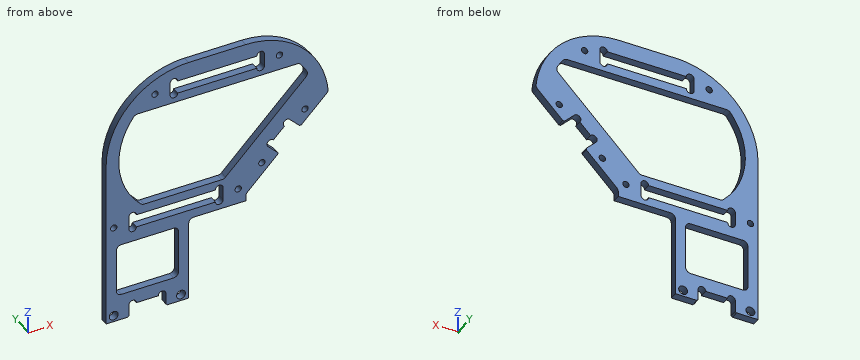
Autodesk Inventor part; units mm, degrees
ref_plane "YZ Plane" through (0, 0, 0) normal (1, 0, 0) x (0, 1, 0)
ref_plane "XZ Plane" through (0, 0, 0) normal (0, 1, 0) x (-1, 0, 0)
ref_plane "XY Plane" through (0, 0, 0) normal (0, 0, 1) x (1, 0, 0)
sketch "Sketch1" plane through (0, 0, 0) normal (0, 1, 0) x (-1, 0, 0)
  line L0 (-16.25, -1.5) -> (16.25, -1.5)
  line L1 (-7.25, -1.5) -> (-7.25, 3.5) construction
  line L2 (-7.25, 3.5) -> (7.25, 3.5) construction
  line L3 (0, 3.5) -> (0, -1.5) construction
  line L4 (7.25, -1.5) -> (7.25, 3.5) construction
  line L5 (-13.25, 1) -> (13.25, 1) construction
  line L6 (-7.3, -1.5) -> (-7.3, 3.5)
  line L7 (-7.3, 3.5) -> (7.3, 3.5)
  arc A0 (-4.3, 3.5) -> (-7.3, 3.5) centre (-5.8, 3.5) ccw
  line L8 (7.3, -1.5) -> (7.3, 3.5)
  arc A1 (7.3, 3.5) -> (4.3, 3.5) centre (5.8, 3.5) ccw
  line L9 (-16.25, -1.5) -> (-16.25, 32)
  line L10 (16.25, -1.5) -> (16.25, 65)
  ellipse E0 centre (-16.25, 65) end of major axis (18.25, 65) minor radius 35 (-16.25, 30) -> (-16.25, 100) ccw construction
  line L11 (-16.25, 30) -> (-16.25, 100) construction
  line L12 (-16.25, 65) -> (18.25, 65) construction
  ellipse E1 centre (-16.25, 65) end of major axis (16.25, 65) minor radius 33 (-16.25, 32) -> (16.25, 65) ccw construction
  line L13 (-16.25, 32) -> (-38.75, 32)
  line L14 (-16.25, 98) -> (-38.75, 98)
  line L15 (-27.5, 98) -> (-27.5, 32) construction
  ellipse E2 centre (-38.75, 65) end of major axis (-73.25, 65) minor radius 35 (-38.75, 100) -> (-38.75, 30) ccw construction
  ellipse E3 centre (-38.75, 65) end of major axis (-71.25, 65) minor radius 33 (-38.75, 98) -> (-71.1715, 67.2921) ccw
  line L16 (-38.75, 30) -> (-16.25, 30) construction
  line L17 (-38.75, 100) -> (-16.25, 100) construction
  line L18 (-10.25, 30) -> (10.25, 30)
  line L19 (12.25, 28) -> (12.25, 11)
  line L20 (10.25, 9) -> (-10.25, 9)
  line L21 (-12.25, 11) -> (-12.25, 28)
  line L22 (-12.25, 30) -> (12.25, 9) construction
  line L23 (12.25, 30) -> (-12.25, 9) construction
  arc A2 (-10.25, 30) -> (-12.25, 28) centre (-10.25, 28) ccw
  arc A3 (-12.25, 11) -> (-10.25, 9) centre (-10.25, 11) ccw
  arc A4 (10.25, 9) -> (12.25, 11) centre (10.25, 11) ccw
  arc A5 (12.25, 28) -> (10.25, 30) centre (10.25, 28) ccw
  line L24 (-38.75, 30) -> (-38.75, 100) construction
  line L25 (-38.75, 32) -> (-38.75, 34.8706)
  line L26 (-38.75, 34.8706) -> (-71.1715, 67.2921)
  line L27 (-62.0208, 45.9792) -> (-108, 0) construction
  line L28 (-108, 0) -> (0, 0) construction
  ellipse E4 centre (-38.75, 65) end of major axis (-71.25, 65) minor radius 33 (-71.1715, 67.2921) -> (-38.75, 32) ccw construction
  ellipse E5 centre (-16.25, 65) end of major axis (16.25, 65) minor radius 33 (16.25, 65) -> (-16.25, 98) ccw
  line L29 (-55, 91.5815) -> (0, 91.5815) construction
  line L30 (0, 91.5815) -> (0, 86.5815) construction
  line L31 (0, 86.5815) -> (-55, 86.5815) construction
  line L32 (-55, 86.5815) -> (-55, 91.5815) construction
  line L33 (-55, 91.5815) -> (0, 86.5815) construction
  line L34 (0, 91.5815) -> (-55, 86.5815) construction
  line L35 (-47.5, 91.5815) -> (-47.5, 96.7815) construction
  line L36 (-47.5, 96.7815) -> (-7.5, 96.7815) construction
  line L37 (-7.5, 96.7815) -> (-7.5, 91.5815) construction
  line L38 (-46, 91.5815) -> (-46, 86.5815) construction
  line L39 (-52, 89.0815) -> (-3, 89.0815) construction
  line L40 (-9, 91.5815) -> (-9, 86.5815) construction
  line L41 (-8.95, 86.5315) -> (-46.05, 86.5315)
  line L42 (-46.05, 86.5315) -> (-46.05, 91.6315)
  line L43 (-46.05, 91.6315) -> (-8.95, 91.6315)
  line L44 (-8.95, 91.6315) -> (-8.95, 86.5315)
  line L45 (-8.95, 86.5315) -> (-46.05, 91.6315) construction
  line L46 (-46.05, 86.5315) -> (-8.95, 91.6315) construction
  arc A6 (-43.05, 91.6315) -> (-46.05, 91.6315) centre (-44.55, 91.6315) ccw
  arc A7 (-46.05, 86.5315) -> (-43.05, 86.5315) centre (-44.55, 86.5315) ccw
  arc A8 (-8.95, 91.6315) -> (-11.95, 91.6315) centre (-10.45, 91.6315) ccw
  arc A9 (-11.95, 86.5315) -> (-8.95, 86.5315) centre (-10.45, 86.5315) ccw
  line L47 (-54.1012, 75.112) -> (-60.6066, 68.6066) construction
  line L48 (-60.6066, 68.6066) -> (-39.3934, 47.3934) construction
  line L49 (-39.3934, 47.3934) -> (-32.888, 53.8988) construction
  line L50 (-32.888, 53.8988) -> (-54.1012, 75.112) construction
  line L51 (-56.0104, 64.0104) -> (-72.2739, 47.747) construction
  line L52 (-72.2739, 47.747) -> (-60.253, 35.7261) construction
  line L53 (-60.253, 35.7261) -> (-43.9896, 51.9896) construction
  line L54 (-60.1823, 56.3029) -> (-56.0104, 60.4749) construction
  line L55 (-56.0104, 60.4749) -> (-47.5251, 51.9896) construction
  line L56 (-47.5251, 51.9896) -> (-51.6971, 47.8177) construction
  line L57 (-60.2177, 56.3383) -> (-56.0458, 60.5102)
  line L58 (-56.0458, 60.5102) -> (-47.4898, 51.9542)
  line L59 (-47.4898, 51.9542) -> (-51.6617, 47.7823)
  arc A10 (-47.4898, 51.9542) -> (-49.6111, 54.0756) centre (-48.5504, 53.0149) ccw
  arc A11 (-53.9244, 58.3889) -> (-56.0458, 60.5102) centre (-54.9851, 59.4496) ccw
  line L60 (-62.0208, 62.9497) -> (-45.0503, 45.9792) construction
  line L61 (-51.7678, 56.2322) -> (-55.3033, 52.6967) construction
  line L62 (-59.5459, 56.9393) -> (-51.0607, 48.4541) construction
  circle A12 centre (-45.0503, 45.9792) radius 2.4 construction
  circle A13 centre (-45.0503, 45.9792) radius 1.25 construction
  line L63 (-65.9099, 63.3033) -> (-62.3744, 66.8388) construction
  line L64 (-44.6967, 42.0901) -> (-41.1612, 45.6256) construction
  line L65 (-29.75, 40.55) -> (7.25, 40.55) construction
  line L66 (7.25, 40.55) -> (7.25, 35.55) construction
  line L67 (7.25, 35.55) -> (-29.75, 35.55) construction
  line L68 (-29.75, 35.55) -> (-29.75, 40.55) construction
  line L69 (-29.75, 40.55) -> (7.25, 35.55) construction
  line L70 (7.25, 40.55) -> (-29.75, 35.55) construction
  line L71 (-35.75, 38.05) -> (13.25, 38.05) construction
  line L72 (-11.25, 40.55) -> (-11.25, 35.55) construction
  line L73 (-38.75, 40.55) -> (-38.75, 35.55) construction
  line L74 (16.25, 40.55) -> (16.25, 35.55) construction
  line L75 (-29.8, 40.6) -> (7.3, 40.6)
  line L76 (7.3, 40.6) -> (7.3, 35.5)
  line L77 (7.3, 35.5) -> (-29.8, 35.5)
  line L78 (-29.8, 35.5) -> (-29.8, 40.6)
  line L79 (-29.8, 40.6) -> (7.3, 35.5) construction
  line L80 (7.3, 40.6) -> (-29.8, 35.5) construction
  arc A14 (4.3, 35.5) -> (7.3, 35.5) centre (5.8, 35.5) ccw
  arc A15 (7.3, 40.6) -> (4.3, 40.6) centre (5.8, 40.6) ccw
  arc A16 (-29.8, 35.5) -> (-26.8, 35.5) centre (-28.3, 35.5) ccw
  arc A17 (-26.8, 40.6) -> (-29.8, 40.6) centre (-28.3, 40.6) ccw
  line L81 (-59.7893, 83.0315) -> (4.7893, 83.0315)
  line L82 (-63.4241, 77.3638) -> (-30.1603, 44.1)
  ellipse E6 centre (-16.25, 65) end of major axis (11.25, 65) minor radius 28.0012 (2.0513, 44.1) -> (11.25, 65) ccw
  ellipse E7 centre (-16.25, 65) end of major axis (11.25, 65) minor radius 28.0012 (11.25, 65) -> (4.7893, 83.0315) ccw
  ellipse E8 centre (-38.75, 65) end of major axis (-66.25, 65) minor radius 28.0012 (-59.7893, 83.0315) -> (-63.4241, 77.3638) ccw
  line L83 (-16.25, 65) -> (8.5857, 86.2852) construction
  line L84 (-30.1603, 44.1) -> (2.0513, 44.1)
  line L85 (-62.0208, 45.9792) -> (-32.844, 9.9488)
  line L86 (-32.844, 9.9488) -> (-98.0512, 75.156)
  line L87 (-98.0512, 75.156) -> (-62.0208, 45.9792)
  line L88 (-38.75, 65) -> (-73.25, 65) construction
  point P0 (0, 1)
  point P1 (0, 19.5)
  point P2 (5.8, 5)
  point P3 (-27.5, 89.0815)
  point P4 (-53.5355, 54.4645)
  point P5 (-50, 58)
  point P6 (-11.25, 38.05)
  point P7 (-11.25, 38.05)
  point P8 (4.3, 3.5)
  point P9 (-53.9244, 58.3889)
  point P10 (-26.8, 35.5)
  point P11 (-26.8, 40.6)
  point P12 (4.3, 40.6)
  point P13 (-11.95, 91.6315)
  point P14 (-11.95, 86.5315)
  point P15 (-43.05, 86.5315)
  point P16 (-10.45, 85.0315)
  point P17 (-28.3, 34)
  point P18 (5.8, 42.1)
  point P19 (-27.5, 89.0815)
  dimension "d0" = 32.5
  dimension "d1" = 9
  dimension "d2" = 6
  dimension "d3" = 1.5
  dimension "d4" = 5
  dimension "d5" = 0.05
  dimension "d7" = 1.5
  dimension "d8" = 70
  dimension "d10" = 100
  dimension "d12" = 2
  dimension "d14" = 2
  dimension "d15" = 22.5
  dimension "d16" = 4
  dimension "d18" = 2
  dimension "d19" = 55
  dimension "d20" = 5
  dimension "d21" = 5.2
  dimension "d22" = 40
  dimension "d24" = 9
  dimension "d25" = 6
  dimension "d26" = 0.05
  dimension "d27" = 0.05
  dimension "d28" = 6
  dimension "d29" = 9.2
  dimension "d30" = 23
  dimension "d31" = 17
  dimension "d32" = 30
  dimension "d33" = 0.05
  dimension "d34" = 5
  dimension "d35" = 6
  dimension "d36" = 2.5
  dimension "d37" = 4.8
  dimension "d38" = 2.5
  dimension "d39" = 1
  dimension "d40" = 50
  dimension "d41" = 58
  dimension "d42" = 45
  dimension "d43" = 30
  dimension "d44" = 9
  dimension "d46" = 5
  dimension "d47" = 6
  dimension "d48" = 9
  dimension "d49" = 0.05
  dimension "d50" = 0.05
  dimension "d54" = 5
  dimension "d56" = 10
  dimension "d59" = 5
  dimension "d61" = 3.55
  dimension "d80" = 55
  dimension "d83" = 2
  dimension "d84" = 2
  dimension "d85" = 168
  dimension "d86" = 24.5
  dimension "d87" = 2
extrude "Extrusion1" add sketch "Sketch1" along normal blind 3 contours L9 L13 L25 L26 L59 A10 L58 A11 L57 E3 L14 E5 L10 L0 L8 A1 L7 A0 L6
hole "Phi3.5" at (13.25, 0, 1) at (-13.25, 0, 1) direction (0, 1, 0) diameter 3.5 end through all
hole "Phi2.5" at (52, 0, 89.0815) at (3, 0, 89.0815) at (62.0208, 0, 62.9497) at (45.0503, 0, 45.9792) at (35.75, 0, 38.05) at (-13.25, 0, 38.05) direction (0, 1, 0) diameter 2.5 end through all
chamfer "C0.5" distance 0.5 angle 45 4 edges at (60.2177, 1.5, 56.3383) (51.6617, 1.5, 47.7823) (7.3, 1.5, -1.5) (-7.3, 1.5, -1.5)
fillet "R2" radius 2 8 edges at (63.4241, 1.5, 77.3638) (59.7893, 1.5, 83.0315) (-4.7893, 1.5, 83.0315) (-2.0513, 1.5, 44.1) (30.1603, 1.5, 44.1) (16.25, 1.5, 32) (38.75, 1.5, 34.8706) (71.1715, 1.5, 67.2921)
equation "\"d14\" = d12"
properties part number "HeadSideFrame" material "CFRP"
The model under review builds one solid part; all positions refer to its coordinate system, in mm. Give positions to 0.01 mm unless a question says otherwise; leave off trailing zeros. Write each loop counter-clockwise with the first axis right and the second up, starting at its lowest first coordinate (ties: lowest second). Pieces come first, ordered by that corner, then holes.
(1) For P1, Ø0.9, axis at x = 24.5, y = 2, coming from the -Z side; P2, Ø1, axis at y = 1.5, z = 32.5, coming from the +X side; P3, Ø0.9, axis at x = 4, y = 1.5, coming from the -Z side, all flat-tipped, find the tip position at first contact; note any pin that passes through.
(2) Consider section C-C, the plane x = 5.8. Give the number of separate pieces and of enclosed holes in the cut face, and give its area (3 significant figures).
(3) To check wall thickness, follow L1, parallel to Z at x = 20, y = 1.8; L2, parallel to Z at x = -6.5, y = 2.3; L3, parallel to Z at x = 53, y = 1.45. State the ranges of each line that lie inside material, in increasing order.
(4) Consider section A-A, the plane z = 16. Give the boundary of the cut face in (x, y).
(5) Consider section B-B, the plane z = 1. Give the boundary of the cut face in (x, y), and give its area (3 significant figures).
Returned:
1. P1: stops at z = 32
1. P2: stops at x = 38.75
1. P3: stops at z = 3.5
2. separate pieces: 4
2. enclosed holes: 0
2. area: 78.6 mm2
3. L1: z = 32 to 35.5, 40.6 to 44.1, 83.03 to 86.53, 91.63 to 98
3. L2: z = 4.83 to 9, 30 to 34.17, 41.93 to 49.27, 80.73 to 88.57
3. L3: z = 57.46 to 66.94, 83.03 to 88.33, 89.83 to 94.66
4. outline: (-16.25, 0) - (-12.25, 0) - (-12.25, 3) - (-16.25, 3) - close; (12.25, 0) - (16.25, 0) - (16.25, 3) - (12.25, 3) - close
5. outline: (-16.25, 0) - (-15, 0) - (-15, 3) - (-16.25, 3) - close; (-11.5, 0) - (-7.3, 0) - (-7.3, 3) - (-11.5, 3) - close; (7.3, 0) - (11.5, 0) - (11.5, 3) - (7.3, 3) - close; (15, 0) - (16.25, 0) - (16.25, 3) - (15, 3) - close
5. area: 32.7 mm2
